The listing builds one solid part. Answer for the finished solid, in the listing's coordinates (mm). Give positions to 0.01 mm unless a question says otherwise; leave off trailing zeros. Order: outer loops, then holes, each group sorted by start corner. A loop starts at its lowest first (then second) coordinate and runs counter-clockwise, first axis right, second up. Notation, with made-up numbers: (69, -29) - (100, -29) arc R30 ccw to (100, -5) - close; hole circle Ø4 at (40.25, -28). An arc over 180 degrees is marked (long way). Use a Markdown table: item, result. Add a question column.
1) The mould has two halves that part along Y. Classify faces 1 (the face through (0.35, -14.84, 1.97)), 2 (the face through (6, 0, 4)), 3 (the face through (0, 15, 2)), 4 (the face through (-1.08, -4.88, 1.97)): released by +Y, released by -Y, zero draft, split by the parting line, or undercut.
2) Find section D-D, the plane y = 13.5. Determine the outline of the cut face in (x, z), plus the area to 3 significant figures.
3) Find section B-B, the plane x = 0. Determine the outline of the cut face in (y, z), plus the area to 3 significant figures.
4) Straight lines are drawn through the part: line 1 (X direction, y = 2, z = 0.8); line 2 (X direction, y = 4, z = 3.15); line 3 (Y direction, x = 1.5, z = 3.45). For each, find the intervals that lie inside material, in ascending order.
5) Find section C-C, the plane z = 1. Determine the outline of the cut face in (x, y).
6) Find section A-A, the plane y = -4. Determine the outline of the cut face in (x, z).
7) A flat-ended cylindrical pin translates along its axis: pin 1 (1 mm diameter, centred on x = -8, z = 3, fed in from -Y). Find the tip coordinate at first contact, or state that the pin passes through.
from build123d import *

# Parameters (mm, degrees)
SKETCH1_R           = 5
BOSS_EXTRUDE1_DEPTH = 4
CUT_EXTRUDE1_DEPTH  = 51


with BuildPart() as part:
    # Sketch1 → Boss-Extrude1 (new body)
    with BuildSketch(Plane.XY):
        with BuildLine():
            Line((-15, 15), (15, 15))
            ThreePointArc((15, 15), (22.071067812, 12.071067812), (25, 5))
            Line((25, 5), (25, -15))
            Line((25, -15), (-25, -15))
            Line((-25, -15), (-25, 5))
            ThreePointArc((-25, 5), (-22.071067812, 12.071067812), (-15, 15))
        make_face()
        Circle(SKETCH1_R, mode=Mode.SUBTRACT)
    extrude(amount=BOSS_EXTRUDE1_DEPTH)

    # Sketch2 → Cut-Extrude1 (cut)
    with BuildSketch(Plane(origin=(25, 0, 0), x_dir=(0, 0, -1), z_dir=(1, 0, 0))):
        with BuildLine():
            Line((-4, -15), (0, -15))
            ThreePointArc((0, -15), (-2, -14.841531007), (-4, -15))
        make_face()
    extrude(amount=-CUT_EXTRUDE1_DEPTH, mode=Mode.SUBTRACT)


solid = part.part
The answers:
| question | item | result |
|---|---|---|
| 1 | face 1 | released by -Y |
| 1 | face 2 | zero draft |
| 1 | face 3 | released by +Y |
| 1 | face 4 | undercut |
| 2 | outline | (-20.27, 0) - (20.27, 0) - (20.27, 4) - (-20.27, 4) - close |
| 2 | area | 162 mm2 |
| 3 | outline | (-15, 0) - (-5, 0) - (-5, 4) - (-15, 4) arc R12.7 cw to start; (5, 0) - (15, 0) - (15, 4) - (5, 4) - close |
| 3 | area | 79.6 mm2 |
| 4 | line 1 | -25 to -4.58, 4.58 to 25 |
| 4 | line 2 | -25 to -3, 3 to 25 |
| 4 | line 3 | -14.92 to -4.77, 4.77 to 15 |
| 5 | outline | (-25, -14.88) - (25, -14.88) - (25, 5) arc R10 ccw to (15, 15) - (-15, 15) arc R10 ccw to (-25, 5) - close; hole circle Ø10 at (0, 0) |
| 6 | outline | (-25, 0) - (-3, 0) - (-3, 4) - (-25, 4) - close; (3, 0) - (25, 0) - (25, 4) - (3, 4) - close |
| 7 | pin 1 | y = -14.93 |
